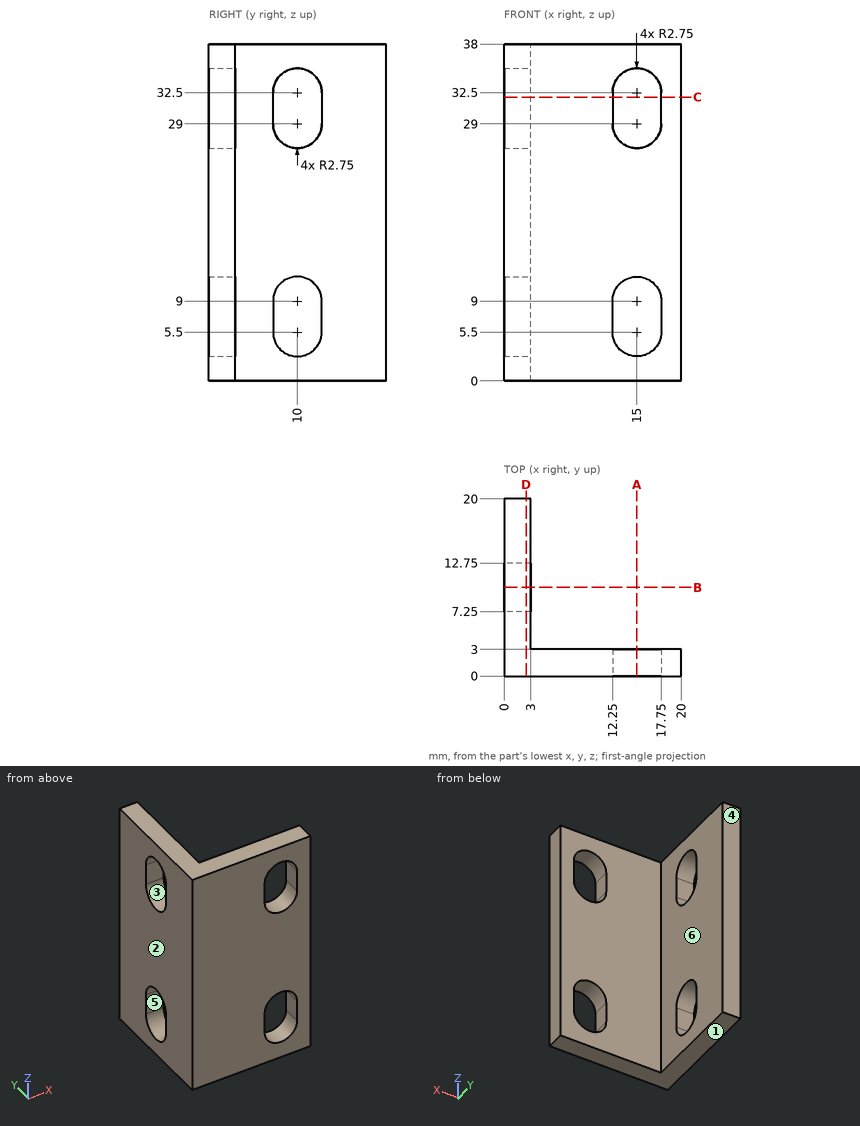
Design review of the part shown in the three views and the two pictorial views. Dimensions are in mm from the part's minimum x, y and z. A direction names the side the tool comes from. Give positions to 0.01 mm unless a question says otherwise; leave off trailing zeros. Loops run counter-clockwise (first coordinate to the right, second up) from the corner with the lowest first, then second, coordinate; pieces in that order, holes last. Notation, with made-up numbers: (-22.5, 81.5) -> (31.5, 81.5) arc R34 cw to (31.5, 116.5) -> close; hole circle Ø10 at (1.5, 80.5). An arc over 180 degrees is marked (long way). One line per question, with ' | ' between items.
1) We need section A-A (x = 15). Write out the cut boundary in (y, z).
Resolved:
outline: (0, 0) -> (3, 0) -> (3, 2.75) -> (0, 2.75) -> close; (0, 11.75) -> (3, 11.75) -> (3, 26.25) -> (0, 26.25) -> close; (0, 35.25) -> (3, 35.25) -> (3, 38) -> (0, 38) -> close
2) For the marked faces 4, 5 and 6, list the 3-axis set-ups (+Z, -Z, +X, -X, +Y, -Y) from which the entire face can be reached by the end or side of a thin tool; tool diameter is ignored.
Resolved:
face 4: +Z, -Z, +X, -X, +Y | face 5: +X, -X | face 6: +Z, -Z, +X, +Y
3) The part is to be moulded in two halves that separate along Z. For the marked faces 1, 2 and 3, say which applies: +Z half, -Z half, draft (parallel to the pull), parting line (faces both ways), or undercut.
Resolved:
face 1: -Z half | face 2: draft | face 3: undercut
4) We need section C-C (z = 32). Write out the cut boundary in (x, y), plus the area to 3 significant figures.
Resolved:
outline: (0, 0) -> (12.25, 0) -> (12.25, 3) -> (3, 3) -> (3, 7.25) -> (0, 7.25) -> close; (0, 12.75) -> (3, 12.75) -> (3, 20) -> (0, 20) -> close; (17.75, 0) -> (20, 0) -> (20, 3) -> (17.75, 3) -> close | area: 78.0 mm2
5) To check wall thickness, follow probe 1 along Z at (x, y) = (2.5, 12); probe 2 along X at (y, z) = (1.25, 6.5); probe 3 along X at (y, z) = (17.75, 34). State the ranges of each line that lie inside material, in increasing order.
Resolved:
probe 1: z = 0 to 3.61, 10.89 to 27.11, 34.39 to 38 | probe 2: x = 0 to 12.25, 17.75 to 20 | probe 3: x = 0 to 3
6) We need section D-D (x = 2.5). Write out the cut boundary in (y, z), plus the area to 3 significant figures.
Resolved:
outline: (0, 0) -> (20, 0) -> (20, 38) -> (0, 38) -> close; hole (7.25, 5.5) arc R2.75 ccw to (12.75, 5.5) -> (12.75, 9) arc R2.75 ccw to (7.25, 9) -> close; hole (7.25, 29) arc R2.75 ccw to (12.75, 29) -> (12.75, 32.5) arc R2.75 ccw to (7.25, 32.5) -> close | area: 674 mm2
7) Insertion check: pin 1 Ø4 at (x, y) = (6, 13) entering from +Z; pin 2 Ø8 at (x, z) = (17.5, 8) entering from +Y. Each pin has a flat end and moves straight along its axis. Give the tip position at first contact, or say it passes through.
Resolved:
pin 1: passes through | pin 2: stops at y = 3
